from build123d import *

# Parameters (mm, degrees)
F0_W     = 46
F0_H     = 145
F0_R     = 2.25
F0_H_2   = 30
F1_DEPTH = 12
F3_DEPTH = 5
F4_R     = 2.15
F5_DEPTH = 25
F6_R     = 3.5
F7_DEPTH = 4
F8_R     = 3.5
F9_DEPTH = 4


with BuildPart() as f1:
    # F0 (on Top) → F1 (new body)
    with BuildSketch(Plane.XY):
        Rectangle(F0_W, F0_H)
        with Locations((-15, -62)):
            Circle(F0_R, mode=Mode.SUBTRACT)
        with Locations((15, -62)):
            Circle(F0_R, mode=Mode.SUBTRACT)
        with Locations((-15, 62)):
            Circle(F0_R, mode=Mode.SUBTRACT)
        with Locations((15, 62)):
            Circle(F0_R, mode=Mode.SUBTRACT)
        with Locations((0, -87.5)):
            Rectangle(F0_W, F0_H_2)
    extrude(amount=F1_DEPTH)

    # F2 (on face) → F3 (cut)
    with BuildSketch(Plane(origin=(0, 0, 0), x_dir=(1, 0, 0), z_dir=(0, 0, -1))):
        Polygon((11.5, -59.979274), (11.5, -64.020726), (15, -66.041452), (18.5, -64.020726), (18.5, -59.979274), (15, -57.958548), align=None)
        Polygon((18.5, 59.979274), (18.5, 64.020726), (15, 66.041452), (11.5, 64.020726), (11.5, 59.979274), (15, 57.958548), align=None)
        Polygon((-11.5, -64.020726), (-11.5, -59.979274), (-15, -57.958548), (-18.5, -59.979274), (-18.5, -64.020726), (-15, -66.041452), align=None)
        Polygon((-11.5, 59.979274), (-11.5, 64.020726), (-15, 66.041452), (-18.5, 64.020726), (-18.5, 59.979274), (-15, 57.958548), align=None)
    extrude(amount=-F3_DEPTH, mode=Mode.SUBTRACT)

    # F4 (on face) → F5 (cut)
    with BuildSketch(Plane.XY.offset(12)):
        with Locations((11, -67)):
            Circle(F4_R)
        with Locations((11, -57)):
            Circle(F4_R)
        with Locations((11, -47)):
            Circle(F4_R)
        with Locations((11, -37)):
            Circle(F4_R)
        with Locations((-11, -67)):
            Circle(F4_R)
        with Locations((-11, -57)):
            Circle(F4_R)
        with Locations((-11, -47)):
            Circle(F4_R)
        with Locations((-11, -37)):
            Circle(F4_R)
        with Locations((11, -27)):
            Circle(F4_R)
        with Locations((-11, -27)):
            Circle(F4_R)
        with Locations((11, -77)):
            Circle(F4_R)
        with Locations((11, -87)):
            Circle(F4_R)
        with Locations((-11, -77)):
            Circle(F4_R)
        with Locations((-11, -87)):
            Circle(F4_R)
    extrude(amount=-F5_DEPTH, mode=Mode.SUBTRACT)

    # F6 (on face) → F7 (cut)
    with BuildSketch(Plane.XY.offset(12)):
        with Locations((11, -67)):
            Circle(F6_R)
        with Locations((11, -57)):
            Circle(F6_R)
        with Locations((11, -47)):
            Circle(F6_R)
        with Locations((11, -37)):
            Circle(F6_R)
        with Locations((11, -27)):
            Circle(F6_R)
        with Locations((-11, -67)):
            Circle(F6_R)
        with Locations((-11, -57)):
            Circle(F6_R)
        with Locations((-11, -47)):
            Circle(F6_R)
        with Locations((-11, -37)):
            Circle(F6_R)
        with Locations((-11, -27)):
            Circle(F6_R)
    extrude(amount=-F7_DEPTH, mode=Mode.SUBTRACT)

    # F8 (on face) → F9 (cut)
    with BuildSketch(Plane.XY.offset(12)):
        with Locations((-11, -77)):
            Circle(F8_R)
        with Locations((-11, -87)):
            Circle(F8_R)
        with Locations((11, -77)):
            Circle(F8_R)
        with Locations((11, -87)):
            Circle(F8_R)
    extrude(amount=-F9_DEPTH, mode=Mode.SUBTRACT)


solid = f1.part
Read the model definition and answer for the solid it produces. Units are mm, in the model's axes. A direction names the side the tool comes from. Give positions to 0.01 mm unless a question says otherwise; leave off trailing zeros. Loops run counter-clockwise (first coordinate to the right, second up) from the corner with the lowest first, then second, coordinate; pieces in that order, holes last. Notation, with made-up numbers: M 44,9.25 L 74,9.25 A19 cw 74,17.25 Z; hole C 61.5,72 d2. An arc over 180 degrees is marked long. Write each question's results on one line, items separated by ' | '.
1. Section A-A on y = -27 is taken. Give the vertices of the cut face in (x, z), plus the area to 3 significant figures.
Values:
outline: M -23,0 L -13.15,0 L -13.15,8 L -14.5,8 L -14.5,12 L -23,12 Z; M -8.85,0 L 8.85,0 L 8.85,8 L 7.5,8 L 7.5,12 L -7.5,12 L -7.5,8 L -8.85,8 Z; M 13.15,0 L 23,0 L 23,12 L 14.5,12 L 14.5,8 L 13.15,8 Z | area: 427 mm^2
2. Section B-B on z = 9.75 is taken. State how many separate pieces and enclosed holes the cut face has, plus the area to 3 significant figures.
Values:
separate pieces: 1 | enclosed holes: 18 | area: 7,450 mm^2
3. A tool of negligible diameter and unlimited length cuts with its end or side. For faces 1 (the face through (-11.5, 62, 2)), 2 (the face through (-10.01, -78.91, 4.06)), 3 (the face through (-13.58, -54.635, 10.028)), from which of +Z, -Z, +X, -X, +Y, -Y can it reach the whole face along a straight path? Write none if from no direction.
Values:
face 1: -Z | face 2: +Z, -Z | face 3: +Z
4. Section C-C on y = -62 is taken. Give the vertices of the cut face in (x, z), plus the area to 3 significant figures.
Values:
outline: M -23,0 L -18.5,0 L -18.5,5 L -17.25,5 L -17.25,12 L -23,12 Z; M -12.75,5 L -11.5,5 L -11.5,0 L 11.5,0 L 11.5,5 L 12.75,5 L 12.75,12 L -12.75,12 Z; M 17.25,5 L 18.5,5 L 18.5,0 L 23,0 L 23,12 L 17.25,12 Z | area: 419 mm^2
5. Straight lines are drawn through the part: line 1 (X direction, y = -62, z = 10.25); line 2 (Y direction, x = 15, z = 9.25); line 3 (Y direction, x = 15, z = 4.5). For each, find the intervals that lie inside material, in ascending order. Write a range as [from, to].
Values:
line 1: x = [-23, -17.25], [-12.75, 12.75], [17.25, 23] | line 2: y = [-102.5, -64.25], [-59.75, 59.75], [64.25, 72.5] | line 3: y = [-102.5, -66.04], [-57.96, 57.96], [66.04, 72.5]
6. Given pin 1 (2.5 mm diameter, centred on x = 15, y = 62, fed in from +Z); pin 2 (2 mm diameter, centred on x = -11.5, y = -38.5, fed in from +Z), each flat-ended and moving along its own axis, determine where each tip first touches the part or whether it passes through.
Values:
pin 1: passes through | pin 2: stops at z = 8
